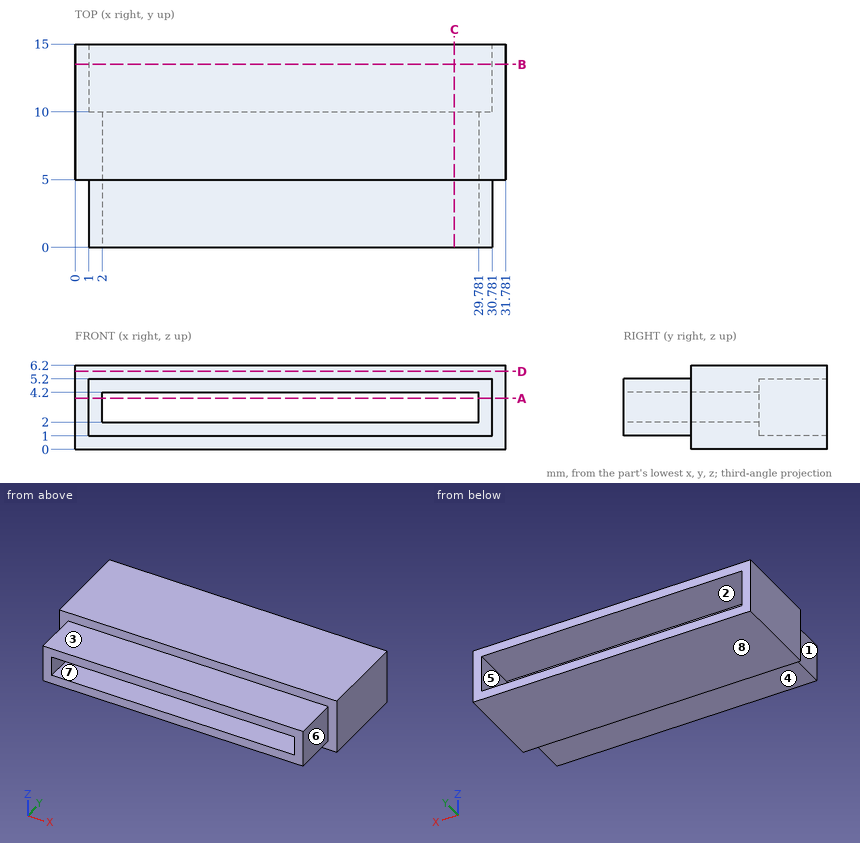
Study the drawing (mm; zero at the part's minimum x, y, z) and answer. A direction names the side the tool comes from. Round coordinates to 2 decimals unless told otherwise and drop trailing zeros. Write each loop counter-clockwise with the first axis right and the second up, starting at its lowest first coordinate (ties: lowest second). Pieces come first, ordered by that corner, then holes.
1) Consider probe 1 along X at (y, z) = (10.25, 2); probe 2 along Z at (x, y) = (2.5, 12.5); probe 3 along X at (y, z) = (2.25, 2.5). Determine where each line is inside the solid, lowest interval first.
2) A cutting plane is placed at D-D on z = 5.75. Determine the outline of the cut face in (x, y), and give its area (3 significant figures).
3) A cutting plane is placed at B-B on y = 13.5. Determine the outline of the cut face in (x, z).
4) A cutting plane is placed at C-C on x = 28. Determine the outline of the cut face in (y, z).
5) Which of the six approach directions +Z, -Z, +X, -X, +Y, -Y give full straight-line access (tool end or side, diameter ignored) to the marked faces 4, 5, 6, 7 and 8?
6) Flat-ended cylindrical pins translate along their axes: P1, Ø1.5, axis at x = 18, y = 3.5, coming from the +Z side; P2, Ø4, axis at x = 17, y = 1.5, coming from the -Z side; P3, Ø3.5, axis at y = 2.5, z = 3.5, coming from the -X side. Find the tip coordinate at first contact, or state that the pin passes through.
7) Determine the mould class of the marked faces 1, 2 and 3 for opening direction X: pulls with the +X half, pulls with the -X half, needs draft (parallel to the pull), parting line crosses it, or undercut.
8) A cutting plane is placed at A-A on z = 3.75. Determine the outline of the cut face in (x, y).
Entries:
1. probe 1: x = 0 to 1, 30.78 to 31.78
1. probe 2: z = 0 to 1, 5.2 to 6.2
1. probe 3: x = 1 to 2, 29.78 to 30.78
2. outline: (0, 5) - (31.78, 5) - (31.78, 15) - (0, 15) - close
2. area: 318 mm2
3. outline: (0, 0) - (31.78, 0) - (31.78, 6.2) - (0, 6.2) - close; hole (1, 1) - (30.78, 1) - (30.78, 5.2) - (1, 5.2) - close
4. outline: (0, 1) - (5, 1) - (5, 0) - (15, 0) - (15, 1) - (10, 1) - (10, 2) - (0, 2) - close; (0, 4.2) - (10, 4.2) - (10, 5.2) - (15, 5.2) - (15, 6.2) - (5, 6.2) - (5, 5.2) - (0, 5.2) - close
5. face 4: -Z, +X, -X, -Y
5. face 5: +Y
5. face 6: +Z, -Z, +X, -Y
5. face 7: +Y, -Y
5. face 8: -Z, +X, -X, +Y, -Y
6. P1: stops at z = 5.2
6. P2: stops at z = 1
6. P3: stops at x = 1
7. face 1: pulls with the -X half
7. face 2: undercut
7. face 3: needs draft
8. outline: (0, 5) - (1, 5) - (1, 0) - (2, 0) - (2, 10) - (1, 10) - (1, 15) - (0, 15) - close; (29.78, 0) - (30.78, 0) - (30.78, 5) - (31.78, 5) - (31.78, 15) - (30.78, 15) - (30.78, 10) - (29.78, 10) - close
